from build123d import *

# Parameters (mm, degrees)
BOSS_EXTRUDE1_DEPTH = 4
SKETCH2_W           = 8.95
SKETCH2_H           = 19.3
SKETCH2_R           = 2.25
BOSS_EXTRUDE2_DEPTH = 4
FILLET1_R           = 10
FILLET2_R           = 4
SKETCH3_W           = 52.4
SKETCH3_H           = 19.3
SKETCH3_R           = 2
BOSS_EXTRUDE3_DEPTH = 4
FILLET3_R           = 10
SKETCH4_W           = 31
SKETCH4_H           = 20.5
CUT_EXTRUDE1_DEPTH  = 10
SKETCH5_W           = 4
SKETCH5_H           = 6
CUT_EXTRUDE2_DEPTH  = 10
FILLET4_R           = 11.55
SKETCH6_W           = 4
SKETCH6_H           = 4
BOSS_EXTRUDE4_DEPTH = 23.3
SKETCH7_R           = 9.5
BOSS_EXTRUDE5_DEPTH = 4
FILLET5_R           = 4


# Some blends are built 0.0001 mm under size
with BuildPart() as part:
    # Sketch1 → Boss-Extrude1 (new body)
    with BuildSketch(Plane(origin=(0, 0, 0), x_dir=(1, 0, 0), z_dir=(0, 1, 0))):
        Polygon((-49, 49.45), (-39, 49.45), (-39, 58.4), (0, 58.4), (0, 0), (-39, 0), (-39, 8.95), (-49, 8.95), align=None)
    extrude(amount=BOSS_EXTRUDE1_DEPTH)

    # Sketch2 → Boss-Extrude2 (add)
    # profile 1 of 2: a face of its own
    with BuildSketch(Plane.ZY.offset(39)):
        with Locations((-4.475, 13.65)):
            Rectangle(SKETCH2_W, SKETCH2_H)
        with Locations((-4.95, 18.55)):
            Circle(SKETCH2_R, mode=Mode.SUBTRACT)
        with Locations((-4.95, 8.55)):
            Circle(SKETCH2_R, mode=Mode.SUBTRACT)
    # profile 2 of 2: a face of its own
    with BuildSketch(Plane.ZY.offset(39)):
        with Locations((-53.925, 13.65)):
            Rectangle(SKETCH2_W, SKETCH2_H)
        with Locations((-54, 18.55)):
            Circle(SKETCH2_R, mode=Mode.SUBTRACT)
        with Locations((-54, 8.55)):
            Circle(SKETCH2_R, mode=Mode.SUBTRACT)
    extrude(amount=-BOSS_EXTRUDE2_DEPTH)

    # Fillet1
    # the kernel refuses this fillet: 10 mm, written as the material it adds along each edge
    with BuildSketch(Plane(origin=(-39, 0, -49.45), x_dir=(-1, 0, 0), z_dir=(0, 1, 0))) as fillet1_piece_1:
        with BuildLine():
            CenterArc((9.944722218, -10), FILLET1_R, 90, 83.97283344)
            Line((0, -8.95), (0, 0))
            Line((0, 0), (9.944722218, 0))
        make_face()
    extrude(amount=4)
    with BuildSketch(Plane(origin=(-39, 0, -8.95), x_dir=(0, 0, 1), z_dir=(0, 1, 0))) as fillet1_piece_2:
        with BuildLine():
            CenterArc((10, -9.944722218), FILLET1_R, 96.02716656, 83.97283344)
            Line((0, -9.944722218), (0, 0))
            Line((0, 0), (8.95, 0))
        make_face()
    extrude(amount=4)

    # Fillet2
    fillet2_edges = [part.edges().sort_by_distance(p)[0] for p in [
        (-37, 23.3, 0),
        (-37, 23.3, -58.4),
    ]]
    fillet(fillet2_edges, radius=FILLET2_R)

    # Sketch3 → Boss-Extrude3 (add)
    with BuildSketch(Plane(origin=(0, 0, 0), x_dir=(0, 0, -1), z_dir=(1, 0, 0))):
        with Locations((32.2, 13.65)):
            Rectangle(SKETCH3_W, SKETCH3_H)
        with Locations((39.95, 13.55)):
            Circle(SKETCH3_R, mode=Mode.SUBTRACT)
    extrude(amount=-BOSS_EXTRUDE3_DEPTH)

    # Fillet3
    fillet3_edges = [part.edges().sort_by_distance(p)[0] for p in [
        (-2, 23.3, -58.4),
    ]]
    fillet(fillet3_edges, radius=FILLET3_R)

    # Sketch4 → Cut-Extrude1 (cut)
    with BuildSketch(Plane(origin=(0, 4, 0), x_dir=(1, 0, 0), z_dir=(0, 1, 0))):
        with Locations((-19.5, 10.25)):
            Rectangle(SKETCH4_W, SKETCH4_H)
    extrude(amount=-CUT_EXTRUDE1_DEPTH, mode=Mode.SUBTRACT)

    # Sketch5 → Cut-Extrude2 (cut)
    with BuildSketch(Plane(origin=(0, 4, 0), x_dir=(1, 0, 0), z_dir=(0, 1, 0))):
        with Locations((-2, 3)):
            Rectangle(SKETCH5_W, SKETCH5_H)
    extrude(amount=-CUT_EXTRUDE2_DEPTH, mode=Mode.SUBTRACT)

    # Fillet4
    fillet4_edges = [part.edges().sort_by_distance(p)[0] for p in [
        (-35, 2, -20.5),
    ]]
    fillet(fillet4_edges, radius=FILLET4_R)

    # Sketch6 → Boss-Extrude4 (add)
    with BuildSketch(Plane(origin=(0, 23.3, 0), x_dir=(1, 0, 0), z_dir=(0, 1, 0))):
        with Locations((2, 8)):
            Rectangle(SKETCH6_W, SKETCH6_H)
    extrude(amount=-BOSS_EXTRUDE4_DEPTH)

    # Sketch7 → Boss-Extrude5 (add)
    with BuildSketch(Plane(origin=(4, 0, 0), x_dir=(0, 0, -1), z_dir=(1, 0, 0))):
        with BuildLine():
            Line((-4.5, 23.3), (10, 23.3))
            Line((10, 23.3), (10, 0))
            Line((10, 0), (-7.7, 0))
            Line((-7.7, 0), (-9, 1.3))
            Line((-9, 1.3), (-17.6, 1.3))
            ThreePointArc((-17.6, 1.3), (-30.2, 13.9), (-17.6, 26.5))
            Line((-17.6, 26.5), (-7.7, 26.5))
            Line((-7.7, 26.5), (-4.5, 23.3))
        make_face()
        with Locations((-17.6, 13.9)):
            Circle(SKETCH7_R, mode=Mode.SUBTRACT)
    extrude(amount=BOSS_EXTRUDE5_DEPTH)

    # Fillet5
    fillet5_edges = [part.edges().sort_by_distance(p)[0] for p in [
        (4, 11.65, -6),
        (0, 11.65, -10),
    ]]
    fillet(fillet5_edges, radius=FILLET5_R)
    fillet5_2_edges = [part.edges().sort_by_distance(p)[0] for p in [
        (-4, 11.65, -6),
        (8, 11.65, -10),
    ]]
    fillet(fillet5_2_edges, radius=FILLET5_R - 0.0001)  # a hair under: the kernel refuses the full size


solid = part.part
Work out the finished part from the listing and answer in its coordinate system (mm). A direction names the side the tool comes from. Give positions to 0.01 mm unless a question says otherwise; leave off trailing zeros. Order: outer loops, then holes, each group sorted by start corner. A loop starts at its lowest first (then second) coordinate and runs counter-clockwise, first axis right, second up. Notation, with made-up numbers: M 83,72.25 L 122,72.25 A14 ccw 122,84.25 Z; hole C 60,49 d8. An arc over 180 degrees is marked long. Return JSON: item names as keys, results as strings.
Q1. Which of the six approach directions +Z, -Z, +X, -X, +Y, -Y give full straight-line access (tool end or side, diameter ignored) to faces 4 (the face through (-37.03, 10.07, -6.61)), 5 (the face through (-14, 2, -20.5)), 6 (the face through (-37, 10, 0)), 7 (the face through (-36.972, 22.097, -1.141)), 8 (the face through (-37, 14, -8.95))?
Answer below:
{"face 4": "-X", "face 5": "+Z, +Y, -Y", "face 6": "+Z, -X, +Y, -Y", "face 7": "+Z, -X, +Y", "face 8": "-X, +Y"}
Q2. The mould has two halves that part along X. Classify faces 1 (the face through (-35, 12, -4)), 2 (the face through (5.97, 21.91, 12.49)), 3 (the face through (6.797, 11.487, -8.859)): pulls with the +X half, pulls with the -X half, needs draft (parallel to the pull), parting line crosses it, or undercut.
Answer below:
{"face 1": "undercut", "face 2": "needs draft", "face 3": "pulls with the +X half"}
Q3. Find section B-B, the plane y = 8.55. State how many separate pieces and enclosed holes the cut face has, and give its area (3 significant figures).
Answer below:
{"separate pieces": "6", "enclosed holes": "0", "area": "354 mm^2"}
Q4. Find the intervals of material crossed by line 1 along Y through (x, z) = (-37.7, -4.95); line 2 along Y through (x, z) = (7.1, 17.6); line 3 along X through (y, z) = (1.25, -5), in increasing order. Write a range as [from, to].
Answer below:
{"line 1": "y = [0, 6.3], [10.8, 16.3], [20.8, 23.3]", "line 2": "y = [1.3, 4.4], [23.4, 26.5]", "line 3": "x = [-40.98, -35], [2.65, 8]"}
Q5. Each of these flat-tipped pins is pushed along its axis until it touches: pin 1 (5 mm diameter, centred on y = 5, z = -44.5, fed in from -X); pin 2 (11.5 mm diameter, centred on y = 10.5, z = -27, fed in from -X); pin 3 (8 mm diameter, centred on y = 15, z = 2, fed in from -X); pin 4 (2.5 mm diameter, centred on y = 15, z = -53, fed in from +X). Where does it stop, or does it pass through?
Answer below:
{"pin 1": "stops at x = -49", "pin 2": "stops at x = -4", "pin 3": "stops at x = -39", "pin 4": "stops at x = 0"}
Q6. Find section A-A, the plane z = -39.95. Write down the section's boundary in (x, y).
Answer below:
{"outline": "M -49,0 L 0,0 L 0,11.55 L -4,11.55 L -4,4 L -49,4 Z; M -4,15.55 L 0,15.55 L 0,23.3 L -4,23.3 Z"}
Q7. Find section D-D, the plane x = -2.5. Write down the section's boundary in (y, z).
Answer below:
{"outline": "M 0,-58.4 L 13.3,-58.4 A10 ccw 23.3,-48.4 L 23.3,-6.88 L 0,-6.88 Z; hole C 13.55,-39.95 d4"}
Q8. Find section C-C, the plane z = 2. Write down the section's boundary in (x, y).
Answer below:
{"outline": "M 4,0 L 8,0 L 8,23.3 L 4,23.3 Z"}
